Design review of the part built by this model. Coordinates are the model's own, in mm. A direction names the side the tool comes from. Round coordinates to 2 decimals unless told otherwise and drop trailing zeros. Write each loop counter-clockwise with the first axis right and the second up, starting at its lowest first coordinate (ties: lowest second). Pieces come first, ordered by that corner, then holes. Notation, with made-up numbers: (-40, 86) -> (-1, 86) arc R8 ccw to (-1, 95) -> close; hole circle Ø6 at (24.25, 47.5). An arc over 180 degrees is marked (long way). Write item = value, one per line. Start each with the question number.
Item 1: Mouldability with a two-part tool opening along Z and no side actions: class faces 5 (the flat face through (-29.842, 4.014, -3.477)), 6 (the flat face through (0, 2, -10)), 7 (the cylindrical face through (-35, 2, 0)) as released by +Z, released by -Z, zero draft, split by the parting line, or undercut.
Item 2: For pin 1 Ø1.5 at (y, z) = (1.5, -2.5) entering from +X; pin 2 Ø2 at (y, z) = (1, -3.5) entering from +X; pin 3 Ø2.5 at (x, z) = (-17, 1.5) entering from +Y; pin 4 Ø2.5 at (x, z) = (0, 4) entering from +Y, all flat-tipped, find the tip position at first contact; note any pin that passes through.
Item 3: Add section C-C, the plane z = -8. State the section outline as (x, y) points.
Item 4: Machinability: for faces 1 (the cylindrical face through (-21.034, 0.986, 0.521)), 2 (the cylindrical face through (35, 2, 0)), 3 (the flat face through (-29.71, 4.01, 3.49)), 4 (the cylindrical face through (-4.5, 4, 0)), which of the approach directions +Z, -Z, +X, -X, +Y, -Y give a long, thin tool a straight path to every point of the face, cutting with its end or side? Answer none if there is none.
Item 5: Add section D-D, the plane x = -27.5. State the section outline as (y, z) points.
Item 6: Add section B-B, the plane x = -16. State the section outline as (y, z) points.
Item 7: To check wall thickness, follow L1, parallel to X at y = 4, z = -4.25; L2, parallel to X at y = 1, z = 0; L3, parallel to Y at x = -24, z = 2.5. State the ranges of each line that lie inside material, in increasing order.
Item 8: Add section A-A, the plane x = 0. State the section outline as (y, z) points.
from build123d import *

# Parameters (mm, degrees)
BOSS_EXTRUDE1_DEPTH = 5
CUT_EXTRUDE4_DEPTH  = 37.742346142
CUT_EXTRUDE5_DEPTH  = 2
SKETCH7_R           = 4
CUT_EXTRUDE6_DEPTH  = 2
CUT_EXTRUDE10_DEPTH = 37.742346142
SKETCH12_R          = 1.75
SKETCH12_R_2        = 1.5
CUT_EXTRUDE11_DEPTH = 37.742346142


with BuildPart() as part:
    # Sketch1 → Boss-Extrude1 (new body)
    with BuildSketch(Plane(origin=(0, 0, 0), x_dir=(1, 0, 0), z_dir=(0, 1, 0))):
        with BuildLine():
            Line((-25, 10), (25, 10))
            ThreePointArc((25, 10), (35, 0), (25, -10))
            Line((25, -10), (-25, -10))
            ThreePointArc((-25, -10), (-35, 0), (-25, 10))
        make_face()
    extrude(amount=BOSS_EXTRUDE1_DEPTH)

    # Sketch5 → Cut-Extrude4 (cut, through all)
    with BuildSketch(Plane(origin=(0, 5, 0), x_dir=(1, 0, 0), z_dir=(0, 1, 0))):
        with BuildLine():
            ThreePointArc((-24, 0), (-24.292893219, 0.707106781), (-25, 1))
            Line((-25, 1), (-25, -1))
            ThreePointArc((-25, -1), (-24.292893219, -0.707106781), (-24, 0))
        make_face()
        with BuildLine():
            Line((-25, -1), (-25, 1))
            ThreePointArc((-25, 1), (-26, 0), (-25, -1))
        make_face()
    extrude(amount=-CUT_EXTRUDE4_DEPTH, mode=Mode.SUBTRACT)

    # Sketch6 → Cut-Extrude5 (cut)
    with BuildSketch(Plane(origin=(0, 5, 0), x_dir=(1, 0, 0), z_dir=(0, 1, 0))):
        with BuildLine():
            Line((-43.5, 2), (-25, 4))
            Line((-25, 4), (-6.5, 2))
            ThreePointArc((-6.5, 2), (-4.5, 0), (-6.5, -2))
            Line((-6.5, -2), (-25, -4))
            Line((-25, -4), (-43.5, -2))
            ThreePointArc((-43.5, -2), (-45.5, 0), (-43.5, 2))
        make_face()
    extrude(amount=-CUT_EXTRUDE5_DEPTH, mode=Mode.SUBTRACT)

    # Sketch7 → Cut-Extrude6 (cut)
    with BuildSketch(Plane.XZ):
        with Locations(Location((-25, 0, 0), (0, 0, 270))):
            Circle(SKETCH7_R)
    extrude(amount=-CUT_EXTRUDE6_DEPTH, mode=Mode.SUBTRACT)

    # Sketch11 → Cut-Extrude10 (cut, through all)
    with BuildSketch(Plane(origin=(0, 5, 0), x_dir=(1, 0, 0), z_dir=(0, 1, 0))):
        with BuildLine():
            ThreePointArc((26.75, 4), (26.237436867, 5.237436867), (25, 5.75))
            Line((25, 5.75), (25, 2.25))
            ThreePointArc((25, 2.25), (26.237436867, 2.762563133), (26.75, 4))
        make_face()
        with BuildLine():
            Line((25, 2.25), (25, 5.75))
            ThreePointArc((25, 5.75), (23.25, 4), (25, 2.25))
        make_face()
        with BuildLine():
            ThreePointArc((26.5, -4), (26.060660172, -2.939339828), (25, -2.5))
            Line((25, -2.5), (25, -5.5))
            ThreePointArc((25, -5.5), (26.060660172, -5.060660172), (26.5, -4))
        make_face()
        with BuildLine():
            Line((25, -5.5), (25, -2.5))
            ThreePointArc((25, -2.5), (23.5, -4), (25, -5.5))
        make_face()
    extrude(amount=-CUT_EXTRUDE10_DEPTH, mode=Mode.SUBTRACT)

    # Sketch12 → Cut-Extrude11 (cut, through all)
    with BuildSketch(Plane(origin=(0, 5, 0), x_dir=(1, 0, 0), z_dir=(0, 1, 0))):
        with Locations(Location((0, 4, 0), (0, 0, 270))):
            Circle(SKETCH12_R)
        with Locations(Location((0, -4, 0), (0, 0, 270))):
            Circle(SKETCH12_R_2)
    extrude(amount=-CUT_EXTRUDE11_DEPTH, mode=Mode.SUBTRACT)


solid = part.part
Result set:
q1.face_5 = undercut
q1.face_6 = released by -Z
q1.face_7 = split by the parting line
q2.pin_1 = 34.85
q2.pin_2 = 34.68
q2.pin_3 = 3
q2.pin_4 = through
q3.outline = (-31, 0) -> (31, 0) -> (31, 5) -> (-31, 5) -> close
q4.face_1 = -Y
q4.face_2 = +X, +Y, -Y
q4.face_3 = +Y
q4.face_4 = -X, +Y
q5.outline = (0, -9.68) -> (5, -9.68) -> (5, -3.73) -> (3, -3.73) -> (3, 3.73) -> (5, 3.73) -> (5, 9.68) -> (0, 9.68) -> (0, 3.12) -> (2, 3.12) -> (2, -3.12) -> (0, -3.12) -> close
q6.outline = (0, -10) -> (5, -10) -> (5, -3.03) -> (3, -3.03) -> (3, 3.03) -> (5, 3.03) -> (5, 10) -> (0, 10) -> close
q7.L1 = -34.05 to -1.73, 1.73 to 23.27, 26.73 to 34.05
q7.L2 = -35 to -29, -21 to 35
q7.L3 = 2 to 3
q8.outline = (0, -10) -> (5, -10) -> (5, -5.75) -> (0, -5.75) -> close; (0, -2.25) -> (5, -2.25) -> (5, 2.5) -> (0, 2.5) -> close; (0, 5.5) -> (5, 5.5) -> (5, 10) -> (0, 10) -> close
